The listing builds one solid part. Answer for the finished solid, in the listing's coordinates (mm). A direction names the side the tool comes from. Coordinates: 2 decimals unless noted, no trailing zeros. Order: outer loops, then holes, each group sorted by start corner. A loop starts at its lowest first (then second) coordinate and runs counter-clockwise, first axis right, second up.
from build123d import *

# Parameters (mm, degrees)
SKETCH1_R           = 5.5
SKETCH1_R_2         = 3.5
BOSS_EXTRUDE1_DEPTH = 10
SKETCH2_R           = 2.5
BOSS_EXTRUDE2_DEPTH = 80
SKETCH3_R           = 3.5
CUT_EXTRUDE1_DEPTH  = 11.0000001


with BuildPart() as part:
    # Sketch1 → Boss-Extrude1 (new body)
    with BuildSketch(Plane.XY):
        Circle(SKETCH1_R)
        Circle(SKETCH1_R_2, mode=Mode.SUBTRACT)
    extrude(amount=BOSS_EXTRUDE1_DEPTH)

    # Sketch2 → Boss-Extrude2 (add)
    with BuildSketch(Plane(origin=(0, 0, 0), x_dir=(1, 0, 0), z_dir=(0, 1, 0))):
        with Locations((0, -5)):
            Circle(SKETCH2_R)
    extrude(amount=BOSS_EXTRUDE2_DEPTH)

    # Sketch3 → Cut-Extrude1 (cut, through all)
    with BuildSketch(Plane.XY.offset(10)):
        Circle(SKETCH3_R)
    extrude(amount=-CUT_EXTRUDE1_DEPTH, mode=Mode.SUBTRACT)


solid = part.part
1) Section A-A (x = 0) is taken. Give the vertices of the cut face in (y, z), then the cut area to 4 significant figures.
2) Each of these flat-tipped pins is pushed along its axis until it touches: P1, Ø5.5, axis at x = 0, y = 0, coming from the -Z side; P2, Ø1, axis at x = 2, y = 54, coming from the -Z side; P3, Ø1.5, axis at y = 23, z = 2.5, coming from the -X side; P4, Ø3, axis at y = 51, z = 5.5, coming from the -X side. Where does it stop, or does it pass through?
3) Section D-D (y = 48) is taken. Give the vertices of the cut face in (x, z), then the cut area to 3 significant figures.
4) Section C-C (z = 5) is taken. Give the vertices of the cut face in (x, y), then the cut area to 3 significant figures.
5) Consider L1, parallel to Y at x = 0, z = 8.75; L2, parallel to Y at x = 0, z = 4.5; L3, parallel to X at y = 76, z = 5. Determine where each line is inside the solid, lowest interval first.
6) A tool of negligible diameter and unlimited length cuts with its end or side. For faces 1 (the face through (-0.33, 41.92, 2.52)), 2 (the face through (4, 0, 0)), from which of +Z, -Z, +X, -X, +Y, -Y can it reach the whole face along a straight path? Write none if from no direction.
7) Section B-B (y = 0) is taken. Give the vertices of the cut face in (x, z), then the cut area to 3 significant figures.
Filled sheet:
1. outline: (-5.5, 0) - (-3.5, 0) - (-3.5, 10) - (-5.5, 10) - close; (3.5, 0) - (5.5, 0) - (5.5, 2.5) - (80, 2.5) - (80, 7.5) - (5.5, 7.5) - (5.5, 10) - (3.5, 10) - close
1. area: 412.5 mm2
2. P1: passes through
2. P2: stops at z = 3
2. P3: stops at x = -1.79
2. P4: stops at x = -2.5
3. outline: circle Ø5 at (0, 5)
3. area: 19.6 mm2
4. outline: (-2.5, 4.9) arc R5.5 ccw (long way) to (2.5, 4.9) - (2.5, 80) - (-2.5, 80) - close; hole circle Ø7 at (0, 0)
4. area: 430 mm2
5. L1: y = -5.5 to -3.5, 3.5 to 5.5
5. L2: y = -5.5 to -3.5, 3.5 to 80
5. L3: x = -2.5 to 2.5
6. face 1: +Y
6. face 2: -Z, +X, -X, +Y, -Y
7. outline: (-5.5, 0) - (-3.5, 0) - (-3.5, 10) - (-5.5, 10) - close; (3.5, 0) - (5.5, 0) - (5.5, 10) - (3.5, 10) - close
7. area: 40.0 mm2
